The model under review builds one solid part; all positions refer to its coordinate system, in mm. Coordinates: 2 decimals unless noted, no trailing zeros. Order: outer loops, then holes, each group sorted by start corner. A loop starts at its lowest first (then second) coordinate and runs counter-clockwise, first axis right, second up. Notation, with made-up numbers: M 21.5,87 L 41.5,87 A18 ccw 41.5,115 Z; hole C 75,74.5 d3. An arc over 180 degrees is marked long. Answer in a Markdown table with one row per item.
from build123d import *

# Parameters (mm, degrees)
SKETCH1_W           = 12.001902846
SKETCH1_H           = 50.8
SKETCH1_R           = 3.175
BOSS_EXTRUDE1_DEPTH = 50.8
SKETCH2_R           = 3.175
SKETCH2_R_2         = 6.35
CUT_EXTRUDE1_DEPTH  = 50.8
CHAMFER1_SIZE       = 0.254


with BuildPart() as part:
    # Sketch1 → Boss-Extrude1 (new body)
    with BuildSketch(Plane(origin=(0, 0, 0), x_dir=(1, 0, 0), z_dir=(0, 1, 0))):
        Rectangle(SKETCH1_W, SKETCH1_H)
        with Locations(Location((0, 19.05, 0), (0, 0, 270))):
            Circle(SKETCH1_R, mode=Mode.SUBTRACT)
        with Locations(Location((0, -19.05, 0), (0, 0, 270))):
            Circle(SKETCH1_R, mode=Mode.SUBTRACT)
    extrude(amount=BOSS_EXTRUDE1_DEPTH)

    # Sketch2 → Cut-Extrude1 (cut)
    with BuildSketch(Plane(origin=(6.000951423, 0, 0), x_dir=(0, 0, -1), z_dir=(1, 0, 0))):
        with Locations((-9.525, 43.18)):
            Circle(SKETCH2_R)
        with Locations((9.525, 43.18)):
            Circle(SKETCH2_R)
        with Locations((0, 27.305)):
            Circle(SKETCH2_R_2)
        with Locations((-9.525, 11.43)):
            Circle(SKETCH2_R)
        with Locations((9.525, 11.43)):
            Circle(SKETCH2_R)
    extrude(amount=-CUT_EXTRUDE1_DEPTH, mode=Mode.SUBTRACT)

    # Chamfer1
    chamfer1_edges = [part.edges().sort_by_distance(p)[0] for p in [
        (6.000951423, 50.8, 0),
        (-6.000951423, 11.43, -6.35),
        (6.000951423, 11.43, -6.35),
        (-6.000951423, 11.43, 12.7),
        (6.000951423, 11.43, 12.7),
        (-6.000951423, 27.305, 6.35),
        (6.000951423, 27.305, 6.35),
        (-6.000951423, 43.18, -6.35),
        (6.000951423, 43.18, -6.35),
        (-6.000951423, 43.18, 12.7),
        (6.000951423, 43.18, 12.7),
        (-6.000951423, 50.8, 0),
        (6.000951423, 0, 0),
        (-6.000951423, 0, 0),
        (-6.000951423, 25.4, -25.4),
        (6.000951423, 25.4, -25.4),
        (6.000951423, 25.4, 25.4),
        (-6.000951423, 25.4, 25.4),
    ]]
    chamfer(chamfer1_edges, length=CHAMFER1_SIZE)


solid = part.part
(1) The part is to be moulded in two halves that separate along Y. For faces 1 (the flat face through (0, 50.8, 0)), 2 (the cylindrical face through (0.08, 12.384, -12.553)), 3 (the flat face through (-6.001, 19, 0)), say which applies: +Y half, -Y half, draft (parallel to the pull), parting line (faces both ways), or undercut.
Report:
| item | result |
|---|---|
| face 1 | +Y half |
| face 2 | undercut |
| face 3 | draft |
(2) To check wall thickness, follow line 1 (Z direction, x = -0.5, y = 7); line 2 (Y direction, x = 0, z = 11); line 3 (Z direction, x = 2.5, y = 22.5). State the ranges of each line that lie inside material, in increasing order. Write a range as [from, to].
Report:
| item | result |
|---|---|
| line 1 | [-25.4, -22.19], [-15.91, 15.91], [22.19, 25.4] |
| line 2 | [0, 8.62], [14.24, 40.37], [45.99, 50.8] |
| line 3 | [-25.4, -21.01], [-17.09, -4.15], [4.15, 17.09], [21.01, 25.4] |
(3) Take a section at D-D (x = -1.5). Write out the cut boundary in (y, z) (3 decimals), then the cut area to 3 significant figures.
Report:
| item | result |
|---|---|
| outline | M 0,-25.4 L 50.8,-25.4 L 50.8,-21.848 L 0,-21.848 Z; M 0,-16.252 L 50.8,-16.252 L 50.8,16.252 L 0,16.252 Z; M 0,21.848 L 50.8,21.848 L 50.8,25.4 L 0,25.4 Z; hole C 11.43,-9.525 d6.35; hole C 11.43,9.525 d6.35; hole C 27.305,0 d12.7; hole C 43.18,-9.525 d6.35; hole C 43.18,9.525 d6.35 |
| area | 1,760 mm^2 |
(4) Take a section at B-B (y = 43.18). Write out the cut boundary in (x, z) (3 decimals), then the cut area to 3 significant figures.
Report:
| item | result |
|---|---|
| outline | M -6.001,-25.146 L -5.747,-25.4 L 5.747,-25.4 L 6.001,-25.146 L 6.001,-12.954 L 5.747,-12.7 L -5.747,-12.7 L -6.001,-12.954 Z; M -6.001,-6.096 L -5.747,-6.35 L 5.747,-6.35 L 6.001,-6.096 L 6.001,6.096 L 5.747,6.35 L -5.747,6.35 L -6.001,6.096 Z; M -6.001,12.954 L -5.747,12.7 L 5.747,12.7 L 6.001,12.954 L 6.001,25.146 L 5.747,25.4 L -5.747,25.4 L -6.001,25.146 Z; hole C 0,-19.05 d6.35; hole C 0,19.05 d6.35 |
| area | 394 mm^2 |
(5) Take a section at C-C (z = 19.05). Write out the cut boundary in (x, y) (3 decimals).
Report:
| item | result |
|---|---|
| outline | M -6.001,0.254 L -5.747,0 L -3.175,0 L -3.175,50.8 L -5.747,50.8 L -6.001,50.546 Z; M 3.175,0 L 5.747,0 L 6.001,0.254 L 6.001,50.546 L 5.747,50.8 L 3.175,50.8 Z |
(6) Take a section at A-A (y = 4.5). Write out the cut boundary in (x, z) (3 decimals), then the cut area to 3 significant figures.
Report:
| item | result |
|---|---|
| outline | M -6.001,-25.146 L -5.747,-25.4 L 5.747,-25.4 L 6.001,-25.146 L 6.001,25.146 L 5.747,25.4 L -5.747,25.4 L -6.001,25.146 Z; hole C 0,-19.05 d6.35; hole C 0,19.05 d6.35 |
| area | 546 mm^2 |
(7) Insertion check: P1, Ø5.5, axis at x = 0, z = 19.05, coming from the +Y side. The pin has a flat end and moves straight along its axis. Give the tip position at first contact, or say it passes through.
Report:
| item | result |
|---|---|
| P1 | through |
